For this review, take the finished solid that the model builds, in its own axes (mm). A direction names the side the tool comes from. Coordinates: 2 decimals unless noted, no trailing zeros. Loops run counter-clockwise (first coordinate to the right, second up) from the corner with the lowest first, then second, coordinate; pieces in that order, holes last.
```python
from build123d import *

# Parameters (mm, degrees)
F0_R     = 12.5
F1_DEPTH = 2
F2_R     = 12.5
F2_R_2   = 11
F3_DEPTH = 10
F4_R     = 2.5
F5_DEPTH = 20


with BuildPart() as f1:
    # F0 (on Front) → F1 (new body)
    with BuildSketch(Plane.XZ):
        Circle(F0_R)
    extrude(amount=F1_DEPTH)

    # F2 (on face) → F3 (join)
    with BuildSketch(Plane.XZ.offset(2)):
        Circle(F2_R)
        Circle(F2_R_2, mode=Mode.SUBTRACT)
    extrude(amount=F3_DEPTH)

    # F4 (on face) → F5 (join)
    with BuildSketch(Plane.XZ.offset(2)):
        Circle(F4_R)
    extrude(amount=F5_DEPTH)


solid = f1.part
```
Q1. Consider section A-A (z = 0). State the section outline as (x, y) points, then the cut area to 3 significant figures.
Q2. Wall thickness on probe 1 along Z at (x, y) = (0, -5); probe 2 along Y at (x, z) = (-8.75, -4.5); probe 3 along Y at (x, z) = (-9.5, -6.5): over which ranges is each line inside the solid? List them lowest first.
Q3. Consider section B-B (y = -2.5). State the section outline as (x, z) points, then the cut area to 3 significant figures.
Q4. Consider section C-C (x = 0). State the section outline as (y, z) points.
Q5. Consider section D-D (y = -17). State the section outline as (x, z) points.
Q6. Machinability: for faces 1 (the face through (-2.38, -6.93, -10.74)), 2 (the face through (0, -22, 0)), which of the approach directions +Z, -Z, +X, -X, +Y, -Y give a long, thin tool a straight path to every point of the face, cutting with its end or side? Answer none if there is none.
Q7. For pin 1 Ø10 at (x, z) = (-9.5, 4.5) entering from -Y; pin 2 Ø1.5 at (y, z) = (-8.5, 1.5) entering from -X; pin 3 Ø2 at (y, z) = (-4.5, 5.5) entering from -X; pin 4 Ø10 at (y, z) = (-14, 4.5) entering from +X, all flat-tipped, find the tip position at first contact; note any pin that passes through.
Q8. The part is to be moulded in two halves that separate along Z. For faces 3 (the face through (-0.54, -11.86, -2.44)), 4 (the face through (5, -12, -10)), 5 (the face through (11.923, -5.916, 3.755)), say which applies: +Z half, -Z half, draft (parallel to the pull), parting line (faces both ways), or undercut.
Model answer:
1. outline: (-12.5, -12) - (-11, -12) - (-11, -2) - (-2.5, -2) - (-2.5, -22) - (2.5, -22) - (2.5, -2) - (11, -2) - (11, -12) - (12.5, -12) - (12.5, 0) - (-12.5, 0) - close
1. area: 180 mm2
2. probe 1: z = -12.5 to -11, -2.5 to 2.5, 11 to 12.5
2. probe 2: y = -2 to 0
2. probe 3: y = -12 to 0
3. outline: circle Ø25 at (0, 0); circle Ø5 at (0, 0); hole circle Ø22 at (0, 0)
3. area: 130 mm2
4. outline: (-22, -2.5) - (-2, -2.5) - (-2, -11) - (-12, -11) - (-12, -12.5) - (0, -12.5) - (0, 12.5) - (-12, 12.5) - (-12, 11) - (-2, 11) - (-2, 2.5) - (-22, 2.5) - close
5. outline: circle Ø5 at (0, 0)
6. face 1: -Y
6. face 2: +Z, -Z, +X, -X, -Y
7. pin 1: stops at y = -12
7. pin 2: stops at x = -12.48
7. pin 3: stops at x = -11.66
7. pin 4: stops at x = 12.5
8. face 3: undercut
8. face 4: draft
8. face 5: parting line
